Work out the finished part from the listing and answer in its coordinate system (mm). A direction names the side the tool comes from. Coordinates: 2 decimals unless noted, no trailing zeros. Order: outer loops, then holes, each group sorted by start corner. A loop starts at its lowest first (then second) coordinate and runs counter-clockwise, first axis right, second up.
```python
from build123d import *

# Parameters (mm, degrees)
F0_W     = 91.5788821876
F0_H     = 24.6932478622
F1_DEPTH = 63.5
F3_DEPTH = 24.6942478622
F4_W     = 91.5788821876
F4_H     = 29.2822020948
F5_DEPTH = 76.2


with BuildPart() as f1:
    # F0 (on Front) → F1 (new body)
    with BuildSketch(Plane.XZ):
        with Locations((5.1525291055, 26.8320306204)):
            Rectangle(F0_W, F0_H)
    extrude(amount=F1_DEPTH)

    # F2 (on face) → F3 (cut, through all)
    with BuildSketch(Plane.XY.offset(39.1786545515)):
        with BuildLine():
            ThreePointArc((-17.3395135884, -13.8349290937), (-19.5607685854, -8.4723451545), (-24.9233525246, -6.2510901575))
            Line((-24.9233525246, -6.2510901575), (-24.9233525246, -21.41876803))
            ThreePointArc((-24.9233525246, -21.41876803), (-19.5607685854, -19.197513033), (-17.3395135884, -13.8349290937))
        make_face()
        with BuildLine():
            Line((36.3587484939, -6.2510901575), (-24.9233525246, -6.2510901575))
            ThreePointArc((-24.9233525246, -6.2510901575), (-19.5607685854, -8.4723451545), (-17.3395135884, -13.8349290937))
            ThreePointArc((-17.3395135884, -13.8349290937), (-19.5607685854, -19.197513033), (-24.9233525246, -21.41876803))
            Line((-24.9233525246, -21.41876803), (36.3587484939, -21.41876803))
            ThreePointArc((36.3587484939, -21.41876803), (29.8547685354, -13.8349290937), (36.3587484939, -6.2510901575))
        make_face()
        with BuildLine():
            Line((-24.9233525246, -21.41876803), (-24.9233525246, -6.2510901575))
            ThreePointArc((-24.9233525246, -6.2510901575), (-32.5071914609, -13.8349290937), (-24.9233525246, -21.41876803))
        make_face()
        with BuildLine():
            ThreePointArc((45.2017359228, -13.8349290937), (42.5236593274, -8.0101321084), (36.3587484939, -6.2510901575))
            Line((36.3587484939, -6.2510901575), (37.5282522291, -6.2510901575))
            Line((37.5282522291, -6.2510901575), (37.5282522291, -21.41876803))
            Line((37.5282522291, -21.41876803), (36.3587484939, -21.41876803))
            ThreePointArc((36.3587484939, -21.41876803), (42.5236593274, -19.659726079), (45.2017359228, -13.8349290937))
        make_face()
        with BuildLine():
            Line((37.5282522291, -6.2510901575), (36.3587484939, -6.2510901575))
            ThreePointArc((36.3587484939, -6.2510901575), (29.8547685354, -13.8349290937), (36.3587484939, -21.41876803))
            Line((36.3587484939, -21.41876803), (37.5282522291, -21.41876803))
            Line((37.5282522291, -21.41876803), (37.5282522291, -6.2510901575))
        make_face()
    extrude(amount=-F3_DEPTH, mode=Mode.SUBTRACT)

    # F4 (on face) → F5 (join)
    with BuildSketch(Plane.XY.offset(39.1786545515)):
        with Locations((5.1525291055, -46.3911010474)):
            Rectangle(F4_W, F4_H)
    extrude(amount=F5_DEPTH)


solid = f1.part
```
1. The part is cut by section B-B (x = 8). Determine the outline of the cut face in (y, z).
2. Flat-ended cylindrical pins translate along their axes: pin 1 (2 mm diameter, centred on x = -7, z = 92.5, fed in from +Y); pin 2 (12.5 mm diameter, centred on x = -1, z = 32.5, fed in from +Y); pin 3 (23 mm diameter, centred on x = 15.5, z = 70.5, fed in from -Y); pin 4 (2 mm diameter, centred on x = 21, y = -62.5, fed in from +Z). Find the tip coordinate at first contact, or state that the pin passes through.
3. The part is cut by section A-A (z = 31.5). Determine the outline of the cut face in (x, y).
4. The part is cut by section D-D (y = -29.5). Determine the outline of the cut face in (x, z).
5. The mould has two halves that part along X. Classify faces 1 (the flat face through (5, -21.419, 27)), 2 (the flat face through (-40.637, -45, 53)), 3 (the flat face through (5, -38, 14.485)): released by +X, released by -X, zero draft, split by the parting line, or undercut.
6. Consider probe 1 along Y at (x, z) = (-3.5, 25); probe 2 along Y at (x, z) = (-7, 77.5); probe 3 along Z at (x, y) = (-26, -28.5). Determine where each line is inside the solid, lowest interval first.
7. For faces 4 (the flat face through (5, -61.032, 77)), 5 (the cylindrical face through (-32.505, -13.668, 27.005)), 6 (the flat face through (5, -23, 39.179)), determine the directions among +Z, -Z, +X, -X, +Y, -Y from which every point of the face is accessible in a straight line to the end or side of a thin tool.
8. The part is cut by section C-C (x = -35). Determine the outline of the cut face in (y, z).
Worked out:
1. outline: (-63.5, 14.49) - (-21.42, 14.49) - (-21.42, 39.18) - (-31.75, 39.18) - (-31.75, 115.38) - (-61.03, 115.38) - (-61.03, 39.18) - (-63.5, 39.18) - close; (-6.25, 14.49) - (0, 14.49) - (0, 39.18) - (-6.25, 39.18) - close
2. pin 1: stops at y = -31.75
2. pin 2: stops at y = 0
2. pin 3: stops at y = -61.03
2. pin 4: stops at z = 39.18
3. outline: (-40.64, -63.5) - (50.94, -63.5) - (50.94, 0) - (-40.64, 0) - close; hole (-24.92, -21.42) - (36.36, -21.42) arc R7.67 ccw (long way) to (36.36, -6.25) - (-24.92, -6.25) arc R7.58 ccw to start
4. outline: (-40.64, 14.49) - (50.94, 14.49) - (50.94, 39.18) - (-40.64, 39.18) - close
5. face 1: undercut
5. face 2: released by -X
5. face 3: zero draft
6. probe 1: y = -63.5 to -21.42, -6.25 to 0
6. probe 2: y = -61.03 to -31.75
6. probe 3: z = 14.49 to 39.18
7. face 4: +Z, +X, -X, -Y
7. face 5: +Z, -Z
7. face 6: +Z, +X, -X, +Y
8. outline: (-63.5, 14.49) - (0, 14.49) - (0, 39.18) - (-31.75, 39.18) - (-31.75, 115.38) - (-61.03, 115.38) - (-61.03, 39.18) - (-63.5, 39.18) - close
